Design review of the part built by this model. Coordinates are the model's own, in mm. Round coordinates to 2 decimals unless told otherwise and drop trailing zeros. Order: outer loops, then holes, each group sorted by start corner. A loop starts at its lowest first (then second) coordinate and runs counter-clockwise, first axis right, second up.
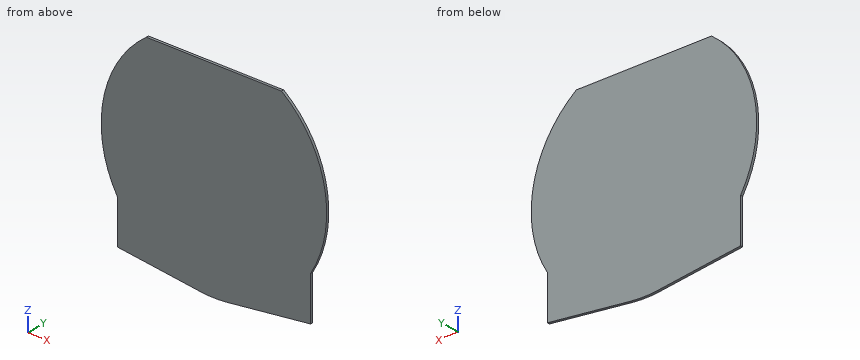
from build123d import *

# Parameters (mm, degrees)
BOSS_EXTRUDE2_DEPTH = 1
MOTOR_SPACING_W     = 154.291365686
MOTOR_SPACING_H     = 35
BOSS_EXTRUDE6_DEPTH = 2
FILLET4_START       = -1
FILLET4_DEPTH       = 2


with BuildPart() as part:
    # Top_lay → Boss-Extrude2 (new, symmetric)
    with BuildSketch(Plane(origin=(0, 0, 0), x_dir=(1, 0, 0), z_dir=(0, 1, 0))):
        with BuildLine():
            Line((-54, -72), (54, -72))
            ThreePointArc((54, -72), (0, 90), (-54, -72))
        make_face()
    extrude(amount=BOSS_EXTRUDE2_DEPTH, both=True)

    # Motor_Spacing → Boss-Extrude6 (add)
    with BuildSketch(Plane(origin=(0, 1, 0), x_dir=(1, 0, 0), z_dir=(0, 1, 0))):
        with Locations((0, 63.828780022)):
            Rectangle(MOTOR_SPACING_W, MOTOR_SPACING_H)
    extrude(amount=-BOSS_EXTRUDE6_DEPTH)

    # Fillet4: read off the stored shape, not the designer's step
    # Fillet4 outline → Fillet4 (add)
    with BuildSketch(Plane(origin=(0, 0, 0), x_dir=(1, 0, 0), z_dir=(0, 1, 0)).offset(FILLET4_START)):
        with BuildLine():
            ThreePointArc((-38.543865143, 81.328780022), (-25.0207268, 86.452086328), (-10.85161032, 89.34339681))
            ThreePointArc((-10.85161032, 89.34339681), (-43.997531602, 85.326865697), (-77.145682843, 81.328780022))
            Line((-77.145682843, 81.328780022), (-38.543865143, 81.328780022))
        make_face()
        with BuildLine():
            ThreePointArc((77.145682843, 81.328780022), (43.997531602, 85.326865697), (10.85161032, 89.34339681))
            ThreePointArc((10.85161032, 89.34339681), (25.0207268, 86.452086328), (38.543865143, 81.328780022))
            Line((38.543865143, 81.328780022), (77.145682843, 81.328780022))
        make_face()
    extrude(amount=FILLET4_DEPTH)


solid = part.part
1) Take a section at A-A on y = -0.7. Give the boundary of the cut face in (x, z), plus the area to 3 significant figures.
Results:
outline: (-77.15, -81.33) arc R60000 cw to (-10.85, -89.34) arc R90 ccw to (10.85, -89.34) arc R60000 cw to (77.15, -81.33) - (77.15, -46.35) arc R90 ccw to (54, 72) - (-54, 72) arc R90 ccw to (-77.15, -46.35) - close
area: 25,500 mm2
2) Clearance check with flat-ended pins moving along their axes: P1, Ø0.6, axis at y = 0, z = -61, coming from the -X side; P2, Ø1, axis at y = 0, z = -56, coming from the +X side. State where each tip first meets the part, or that it passes through.
Results:
P1: stops at x = -77.15
P2: stops at x = 77.15
3) Take a section at C-C on z = -23. Give the boundary of the cut face in (x, y), plus the area to 3 significant figures.
Results:
outline: (-87.01, -1) - (87.01, -1) - (87.01, 1) - (-87.01, 1) - close
area: 348 mm2
4) To check wall thickness, follow line 1 along X through (y, z) = (0.65, -1.5); line 2 along X through (y, z) = (0.75, -46.5); line 3 along Z through (x, y) = (-8, -0.2). State the ranges of each line that lie inside material, in increasing order.
Results:
line 1: x = -89.99 to 89.99
line 2: x = -77.15 to 77.15
line 3: z = -89.64 to 72
5) Take a section at B-B on x = 41. Give the boundary of the cut face in (y, z), plus the area to 3 significant figures.
Results:
outline: (-1, -85.69) - (1, -85.69) - (1, 72) - (-1, 72) - close
area: 315 mm2
